```python
from build123d import *

# Parameters (mm, degrees)
SKETCH2_W           = 40
SKETCH2_H           = 44
BOSS_EXTRUDE1_DEPTH = 4
SKETCH4_W           = 40
SKETCH4_H           = 4
BOSS_EXTRUDE2_DEPTH = 40
SKETCH5_R           = 1.7
CUT_EXTRUDE1_DEPTH  = 72.665891469
SKETCH8_R           = 1.7
CUT_EXTRUDE4_DEPTH  = 72.665891469
FILLET2_R           = 1


with BuildPart() as part:
    # Sketch2 → Boss-Extrude1 (new body)
    with BuildSketch(Plane.XY):
        with Locations((20, 22)):
            Rectangle(SKETCH2_W, SKETCH2_H)
    extrude(amount=BOSS_EXTRUDE1_DEPTH)

    # Sketch4 → Boss-Extrude2 (add)
    with BuildSketch(Plane.XY.offset(4)):
        with Locations((20, 2)):
            Rectangle(SKETCH4_W, SKETCH4_H)
    extrude(amount=BOSS_EXTRUDE2_DEPTH)

    # Sketch5 → Cut-Extrude1 (cut, through all)
    with BuildSketch(Plane.XY.offset(4)):
        with BuildLine():
            ThreePointArc((29, 24), (26.363961031, 30.363961031), (20, 33))
            Line((20, 33), (20, 15))
            ThreePointArc((20, 15), (26.363961031, 17.636038969), (29, 24))
        make_face()
        with BuildLine():
            Line((20, 15), (20, 33))
            ThreePointArc((20, 33), (11, 24), (20, 15))
        make_face()
        with Locations((9, 24)):
            Circle(SKETCH5_R)
        with Locations((20, 35)):
            Circle(SKETCH5_R)
        with Locations((31, 24)):
            Circle(SKETCH5_R)
        with Locations((20, 13)):
            Circle(SKETCH5_R)
    extrude(amount=-CUT_EXTRUDE1_DEPTH, mode=Mode.SUBTRACT)

    # Sketch8 → Cut-Extrude4 (cut, through all)
    with BuildSketch(Plane(origin=(0, 4, 0), x_dir=(1, 0, 0), z_dir=(0, 1, 0))):
        with Locations(Location((5, -9, 0), (0, 0, 270))):
            Circle(SKETCH8_R)
        with Locations(Location((35, -9, 0), (0, 0, 270))):
            Circle(SKETCH8_R)
        with Locations(Location((35, -39, 0), (0, 0, 270))):
            Circle(SKETCH8_R)
        with Locations(Location((5, -39, 0), (0, 0, 270))):
            Circle(SKETCH8_R)
    extrude(amount=-CUT_EXTRUDE4_DEPTH, mode=Mode.SUBTRACT)

    # Fillet2
    fillet2_edges = [part.edges().sort_by_distance(p)[0] for p in [
        (40, 24, 4),
        (0, 4, 24),
        (20, 44, 4),
        (20, 4, 4),
        (40, 4, 24),
        (0, 2, 44),
        (20, 0, 44),
        (40, 2, 44),
        (20, 4, 44),
        (0, 24, 4),
        (20, 44, 0),
        (40, 22, 0),
        (20, 0, 0),
        (0, 22, 0),
        (0, 44, 2),
        (40, 44, 2),
        (40, 0, 22),
        (0, 0, 22),
    ]]
    fillet(fillet2_edges, radius=FILLET2_R)


solid = part.part
```
The model under review builds one solid part; all positions refer to its coordinate system, in mm. A direction names the side the tool comes from. Give positions to 0.01 mm unless a question says otherwise; leave off trailing zeros. Write each loop counter-clockwise with the first axis right and the second up, starting at its lowest first coordinate (ties: lowest second). Pieces come first, ordered by that corner, then holes. Notation, with made-up numbers: (3.5, -24.75) - (41.5, -24.75) arc R31 cw to (41.5, 0.25) - close; hole circle Ø4 at (46, 58). An arc over 180 degrees is marked (long way). Answer in a Markdown table with one row per item. Add a question column.
1. We need section B-B on x = 31. Write out the cut boundary in (y, z), then the cut area to 3 significant figures.
2. We need section C-C on y = 35. Write out the cut boundary in (x, z).
3. We need section A-A on z = 9. Write out the cut boundary in (x, y), then the cut area to 3 significant figures.
4. Draft analysis for pull direction Z (two halves, no side actions). For faces 1 (the flat face through (20, 2, 44)), 2 (the flat face through (20, 4, 24)), 3 (the cylindrical face through (33.34, 2.03, 38.63)), state which applies: +Z half, -Z half, draft (parallel to the pull), parting line (faces both ways), or undercut.
5. Insertion check: P1, Ø2, axis at x = 9, y = 24, coming from the +Z side; P2, Ø8, axis at x = 32, z = 25, coming from the +Y side; P3, Ø4.5, axis at x = 20, y = 13, coming from the +Z side. Each pin has a flat end and moves straight along its axis. Give the tip position at first contact, or say it passes through.
6. Tool access review of faces 4 (the flat face through (40, 13, 2)), 5 (the flat face through (11, 28, 4)): name each direction out of +Z, -Z, +X, -X, +Y, -Y from which nothing blocks a thin tool from reaching the whole face with its end or side.
7. We need section D-D on y = 7. Write out the cut boundary in (x, z).
8. Wall thickness on line 1 along X through (y, z) = (2.3, 39); line 2 along Y through (x, z) = (20, 3); line 3 along Y through (x, z) = (31, 24): over which ranges is each line inside the solid? List them lowest first. Write a range as [from, to].
Ans:
| question | item | result |
|---|---|---|
| 1 | outline | (0, 1) arc R1 ccw to (1, 0) - (22.3, 0) - (22.3, 4) - (5, 4) arc R1 cw to (4, 5) - (4, 43) arc R1 ccw to (3, 44) - (1, 44) arc R1 ccw to (0, 43) - close; (25.7, 0) - (43, 0) arc R1 ccw to (44, 1) - (44, 3) arc R1 ccw to (43, 4) - (25.7, 4) - close |
| 1 | area | 322 mm^2 |
| 2 | outline | (0, 1) arc R1 ccw to (1, 0) - (18.3, 0) - (18.3, 4) - (1, 4) arc R1 ccw to (0, 3) - close; (21.7, 0) - (39, 0) arc R1 ccw to (40, 1) - (40, 3) arc R1 ccw to (39, 4) - (21.7, 4) - close |
| 3 | outline | (0, 1) arc R1 ccw to (1, 0) - (3.3, 0) - (3.3, 4) - (1, 4) arc R1 ccw to (0, 3) - close; (6.7, 0) - (33.3, 0) - (33.3, 4) - (6.7, 4) - close; (36.7, 0) - (39, 0) arc R1 ccw to (40, 1) - (40, 3) arc R1 ccw to (39, 4) - (36.7, 4) - close |
| 3 | area | 132 mm^2 |
| 4 | face 1 | +Z half |
| 4 | face 2 | draft |
| 4 | face 3 | undercut |
| 5 | P1 | passes through |
| 5 | P2 | stops at y = 4 |
| 5 | P3 | stops at z = 4 |
| 6 | face 4 | +Z, -Z, +X, +Y, -Y |
| 6 | face 5 | +Z, +X, -X, +Y |
| 7 | outline | (0, 1) arc R1 ccw to (1, 0) - (39, 0) arc R1 ccw to (40, 1) - (40, 3) arc R1 ccw to (39, 4) - (1, 4) arc R1 ccw to (0, 3) - close |
| 8 | line 1 | x = [0, 3.3], [6.7, 33.3], [36.7, 40] |
| 8 | line 2 | y = [0, 11.3], [14.7, 15], [33, 33.3], [36.7, 44] |
| 8 | line 3 | y = [0, 4] |
